```python
from build123d import *

# Parameters (mm, degrees)
CROQUIS4_W                = 13
CROQUIS4_H                = 11.3
SALIENTE_EXTRUIR1_DEPTH   = 161
CROQUIS5_W                = 151
CROQUIS5_H                = 3.5
CORTAR_EXTRUIR1_DEPTH     = 6.3
SALIENTE_EXTRUIR3_DEPTH   = 8
CROQUIS9_R                = 2.5
CORTAR_EXTRUIR3_DEPTH     = 179.518038304
SIMETR_A8_COPY_1_DEPTH    = 8
SIMETR_A8_COPY_2_SKETCH_R = 2.5
SIMETR_A8_COPY_2_DEPTH    = 179.518038304
CROQUIS10_R               = 2.5
CORTAR_EXTRUIR4_DEPTH     = 179.518038304
MATRIZL1_COUNT            = 3
MATRIZL1_PITCH            = 40.5
CROQUIS11_W               = 61.925542409
CROQUIS11_H               = 21.407853528
CORTAR_EXTRUIR5_DEPTH     = 167.107465215


with BuildPart() as part:
    # Barrer1: sweep along a path in Croquis3
    with BuildLine(Plane(origin=(0, 0, 0), x_dir=(1, 0, 0), z_dir=(0, 1, 0))) as barrer1_path:
        Line((0, 0), (0, -37))
    # Croquis1 → Barrer1 (sweep)
    with BuildSketch(Plane.XY):
        Polygon((0, 0), (0, 11.3), (13, 11.3), (13, 6.3), (5, 6.3), (5, 0), align=None)
    barrer1 = sweep(path=barrer1_path.line)

    # Croquis4 → Saliente-Extruir1 (add)
    with BuildSketch(Plane.ZY):
        with Locations((43.5, 5.65)):
            Rectangle(CROQUIS4_W, CROQUIS4_H)
    extrude(amount=-SALIENTE_EXTRUIR1_DEPTH)

    # Simetría5: Barrer1 across plane
    add(barrer1.mirror(Plane.ZY.offset(-80.5)))

    # Croquis5 → Cortar-Extruir1 (cut)
    with BuildSketch(Plane.XZ):
        with Locations((80.5, 38.75)):
            Rectangle(CROQUIS5_W, CROQUIS5_H)
    extrude(amount=-CORTAR_EXTRUIR1_DEPTH, mode=Mode.SUBTRACT)

    # Croquis8 → Saliente-Extruir3 (add)
    with BuildSketch(Plane.XZ):
        with BuildLine():
            Line((161, 46), (165, 46))
            ThreePointArc((165, 46), (171, 40), (165, 34))
            Line((165, 34), (161, 34))
            Line((161, 34), (161, 46))
        make_face()
    saliente_extruir3 = extrude(amount=-SALIENTE_EXTRUIR3_DEPTH)

    # Croquis9 → Cortar-Extruir3 (cut, through all)
    with BuildSketch(Plane.XZ):
        with Locations((165, 40)):
            Circle(CROQUIS9_R)
    cortar_extruir3 = extrude(amount=-CORTAR_EXTRUIR3_DEPTH, mode=Mode.SUBTRACT)

    # Simetría7: Saliente-Extruir3, Cortar-Extruir3 across plane
    add(saliente_extruir3.mirror(Plane(origin=(0, 0, 24), x_dir=(1, 0, 0), z_dir=(0, 0, -1))))
    add(cortar_extruir3.mirror(Plane(origin=(0, 0, 24), x_dir=(1, 0, 0), z_dir=(0, 0, -1))), mode=Mode.SUBTRACT)

    # Simetría8: Saliente-Extruir3, Cortar-Extruir3 across plane
    add(saliente_extruir3.mirror(Plane.ZY.offset(-80.5)))
    add(cortar_extruir3.mirror(Plane.ZY.offset(-80.5)), mode=Mode.SUBTRACT)

    # Simetría8 copy 1 sketch → Simetría8 copy 1 (add)
    with BuildSketch(Plane(origin=(161, 0, 48), x_dir=(-1, 0, 0), z_dir=(0, -1, 0))):
        with BuildLine():
            Line((161, 46), (165, 46))
            ThreePointArc((165, 46), (171, 40), (165, 34))
            Line((165, 34), (161, 34))
            Line((161, 34), (161, 46))
        make_face()
    extrude(amount=-SIMETR_A8_COPY_1_DEPTH)

    # Simetría8 copy 2 sketch → Simetría8 copy 2 (cut, through all)
    with BuildSketch(Plane(origin=(161, 0, 48), x_dir=(-1, 0, 0), z_dir=(0, -1, 0))):
        with Locations((165, 40)):
            Circle(SIMETR_A8_COPY_2_SKETCH_R)
    extrude(amount=-SIMETR_A8_COPY_2_DEPTH, mode=Mode.SUBTRACT)

    # Croquis10 → Cortar-Extruir4 (cut, through all)
    with BuildSketch(Plane(origin=(0, 11.3, 0), x_dir=(1, 0, 0), z_dir=(0, 1, 0))):
        with Locations(Location((121, -45.25, 0), (0, 0, 270))):
            Circle(CROQUIS10_R)
    cortar_extruir4 = extrude(amount=-CORTAR_EXTRUIR4_DEPTH, mode=Mode.SUBTRACT)

    # MatrizL1: Cortar-Extruir4 ×3
    with Locations(*[(-i * MATRIZL1_PITCH, 0, 0) for i in range(1, MATRIZL1_COUNT)]):
        add(cortar_extruir4, mode=Mode.SUBTRACT)

    # Croquis11 → Cortar-Extruir5 (cut, through all)
    with BuildSketch(Plane.ZY.offset(-148)):
        with Locations((24.861164112, 5.775)):
            Rectangle(CROQUIS11_W, CROQUIS11_H)
    extrude(amount=CORTAR_EXTRUIR5_DEPTH, mode=Mode.SUBTRACT)


solid = part.part
```
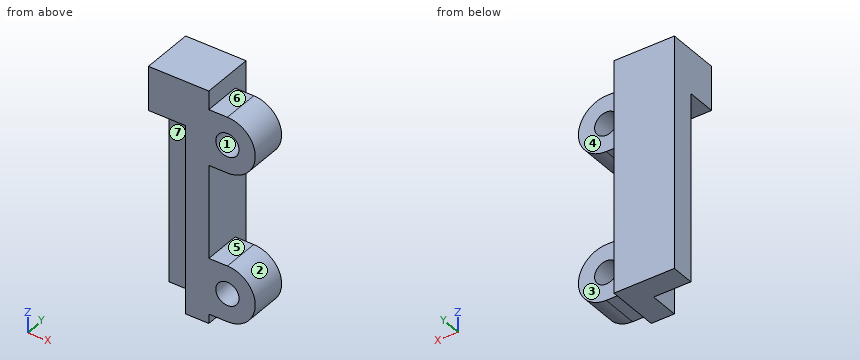
For this review, take the finished solid that the model builds, in its own axes (mm). Face numbers are marked on the shaded views. A direction names the side the tool comes from. Coordinates: 2 decimals unless noted, no trailing zeros. Loops run counter-clockwise (first coordinate to the right, second up) from the corner with the lowest first, then second, coordinate; pieces in that order, holes last. Notation, with made-up numbers: (68.5, 19) - (103.5, 19) arc R36 ccw to (103.5, 55) - close; hole circle Ø4 at (-36, -17.5). An arc over 180 degrees is marked (long way). Use one line per item in the form item = value. Start each with the question number.
1) To check wall thickness, follow probe 1 along Z at (x, y) = (165, 3.75); probe 2 along Z at (x, y) = (163.75, 3.25); probe 3 along Y at (x, z) = (168.25, 3). State the ranges of each line that lie inside material, in increasing order. Write a range as from..to.
2) Take a section at C-C (x = 155.5). State the section outline as (y, z) points.
3) For pin 1 (1.2 mm diameter, centred on x = 163.5, y = 5, fed in from +Z); pin 2 (1.9 mm diameter, centred on x = 151.5, y = 4.5, fed in from -Z); pin 3 (5 mm diameter, centred on x = 165.5, z = 42.5, fed in from +Y), all flat-tipped, find the tip position at first contact; note any pin that passes through.
4) Take a section at A-A (z = 40). State the section outline as (x, y) points.
5) Take a section at D-D (y = 8.5). State the section outline as (x, z) points, plus the area to 3 significant figures.
6) For the marked faces 4, 5, 6 and 7, list the 3-axis set-ups (+Z, -Z, +X, -X, +Y, -Y) from which the entire face can be reached by the end or side of a thin tool; tool diameter is ignored.
7) Draft analysis for pull direction X (two halves, no side actions). For the marked faces 1, 2 and 3, state which applies: released by +X, released by -X, zero draft, split by the parting line, or undercut.
8) Take a section at B-B (y = 5). State the section outline as (x, z) points.
From the geometry:
q1.probe_1 = 2..5.5, 10.5..14, 34..37.5, 42.5..46
q1.probe_2 = 2..5.83, 10.17..14, 34..37.83, 42.17..46
q1.probe_3 = 0..8
q2.outline = (0, 40.5) - (6.3, 40.5) - (6.3, 0) - (11.3, 0) - (11.3, 50) - (0, 50) - close
q3.pin_1 = 46
q3.pin_2 = 40.5
q3.pin_3 = 8
q4.outline = (148, 6.3) - (156, 6.3) - (156, 0) - (162.5, 0) - (162.5, 8) - (161, 8) - (161, 11.3) - (148, 11.3) - close; (167.5, 0) - (171, 0) - (171, 8) - (167.5, 8) - close
q5.outline = (148, 0) - (161, 0) - (161, 50) - (148, 50) - close
q5.area = 650 mm2
q6.face_4 = +Z, -Z, +X, +Y
q6.face_5 = +X, +Y, -Y
q6.face_6 = +Z, +X, +Y, -Y
q6.face_7 = -Z, -X, -Y
q7.face_1 = undercut
q7.face_2 = released by +X
q7.face_3 = zero draft
q8.outline = (148, 40.5) - (156, 40.5) - (156, 0) - (161, 0) - (161, 2) - (165, 2) arc R6 ccw to (165, 14) - (161, 14) - (161, 34) - (165, 34) arc R6 ccw to (165, 46) - (161, 46) - (161, 50) - (148, 50) - close; hole circle Ø5 at (165, 8); hole circle Ø5 at (165, 40)
